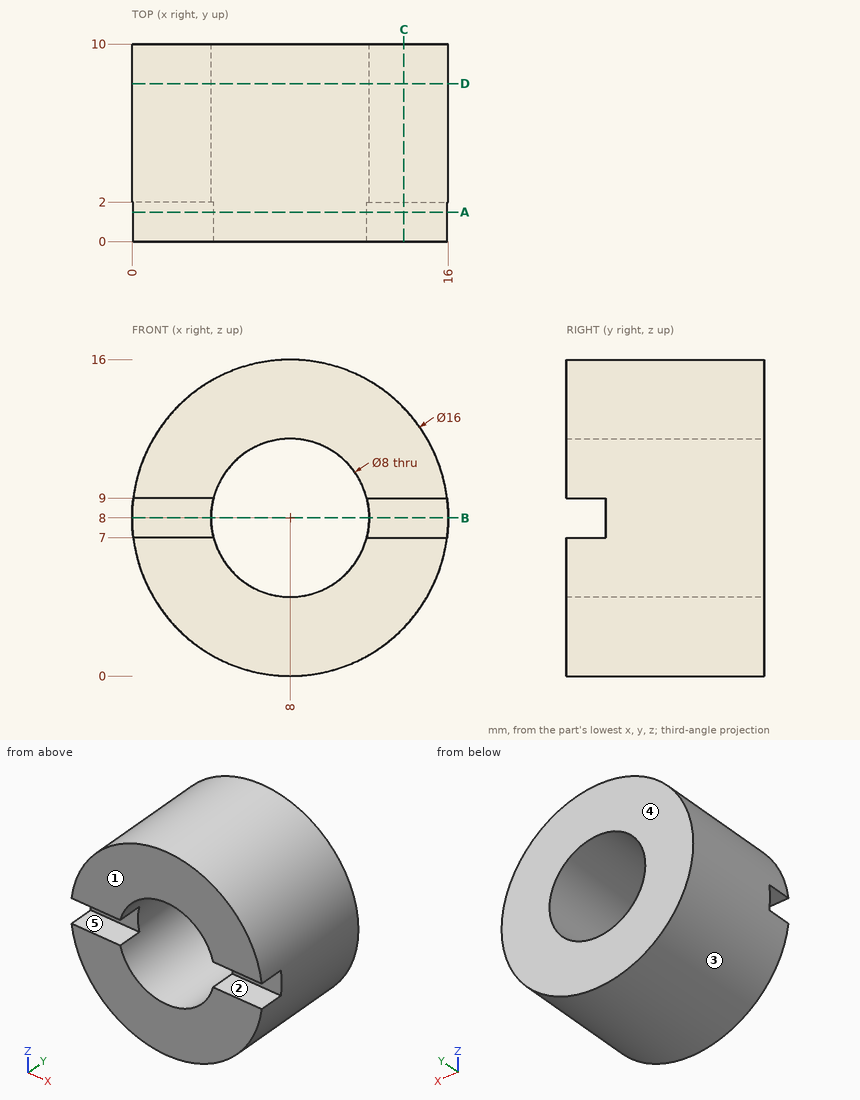
The drawing under review shows one solid part. Ordinate dimensions are in mm from its lowest x, y, z. A direction names the side the tool comes from. Round coordinates to 2 decimals unless told otherwise and drop trailing zeros. Write each loop counter-clockwise with the first axis right and the second up, starting at its lowest first coordinate (ties: lowest second). Pieces come first, ordered by that corner, then holes.
(1) We need section B-B on z = 8. Give the boundary of the cut face in (x, y).
(2) We need section A-A on y = 1.5. Give the boundary of the cut face in (x, z).
(3) We need section C-C on x = 13.75. Give the boundary of the cut face in (y, z).
(4) Wall thickness on L1, parallel to X at y = 3, z = 8; L2, parallel to Y at x = 15, z = 8.25: over which ranges is each line inside the solid? List them lowest first.
(5) Insertion check: pin 1 (1.5 mm diameter, centred on x = 13.5, y = 8, fed in from +Z); pin 2 (0.6 mm diameter, centred on x = 1.5, y = 0.5, fed in from +Z); pin 3 (1.6 mm diameter, centred on x = 13.5, y = 1.5, fed in from +Z). Each pin has a flat end and moves straight along its axis. Give the tip position at first contact, or say it passes through.
(6) Mouldability with a two-part tool opening along Z and no side actions: class the marked faces 1, 2 and 3 as +Z half, -Z half, draft (parallel to the pull), parting line (faces both ways), or undercut.
(7) We need section D-D on y = 8. Give the boundary of the cut face in (x, z), and give its area (3 significant figures).
(8) Machinability: for the marked faces 4 and 5, which of the approach directions +Z, -Z, +X, -X, +Y, -Y give a long, thin tool a straight path to every point of the face, cutting with its end or side? Answer none if there is none.
Findings below:
1. outline: (0, 2) - (4, 2) - (4, 10) - (0, 10) - close; (12, 2) - (16, 2) - (16, 10) - (12, 10) - close
2. outline: (0.06, 7) arc R8 ccw to (15.94, 7) - (11.87, 7) arc R4 cw to (4.13, 7) - close; (0.06, 9) - (4.13, 9) arc R4 cw to (11.87, 9) - (15.94, 9) arc R8 ccw to start
3. outline: (0, 2.44) - (10, 2.44) - (10, 13.56) - (0, 13.56) - (0, 9) - (2, 9) - (2, 7) - (0, 7) - close
4. L1: x = 0 to 4, 12 to 16
4. L2: y = 2 to 10
5. pin 1: stops at z = 14.44
5. pin 2: stops at z = 13.06
5. pin 3: stops at z = 14.47
6. face 1: draft
6. face 2: undercut
6. face 3: parting line
7. outline: circle Ø16 at (8, 8); hole circle Ø8 at (8, 8)
7. area: 151 mm2
8. face 4: +Z, -Z, +X, -X, +Y
8. face 5: +X, -X, -Y
